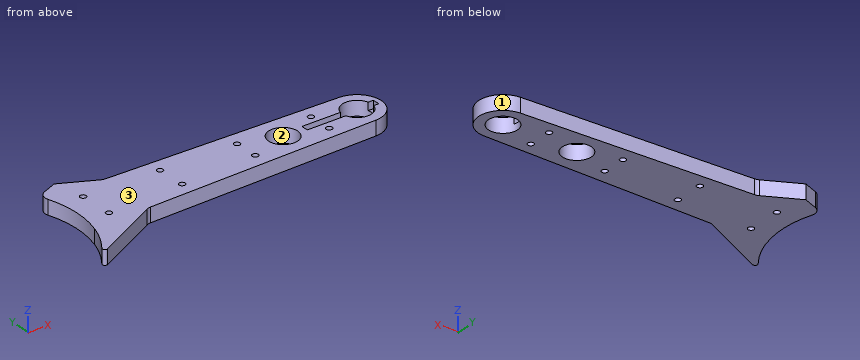
```python
from build123d import *

# Parameters (mm, degrees)
SKETCH1_R                = 13.5
SKETCH1_R_2              = 3
BOSS_EXTRUDE1_DEPTH      = 3
M2_CLEARANCE_HOLE1_D     = 2.4
M2_CLEARANCE_HOLE1_DEPTH = 11.5
CIRPATTERN1_COUNT        = 12
TROU_TARAUD_M1_61_D      = 1.25
ESQUISSE1_R              = 21
ENL_V_MAT_EXTRU_1_DEPTH  = 4
ESQUISSE2_R              = 0.625
ENL_V_MAT_EXTRU_2_DEPTH  = 4
ESQUISSE4_W              = 15
ESQUISSE4_H              = 1.5
ENL_V_MAT_EXTRU_3_DEPTH  = 1.6
ESQUISSE5_R              = 0.625
ENL_V_MAT_EXTRU_4_DEPTH  = 10
BOSS_EXTRU_3_DEPTH       = 3
CONG_2_R                 = 2
CONG_3_R                 = 2
CONG_4_R                 = 0.5


with BuildPart() as part:
    # Sketch1 → Boss-Extrude1 (new body)
    with BuildSketch(Plane.XY):
        with BuildLine():
            Line((18.384776311, 6.5), (80.121567237, 4.998521922))
            ThreePointArc((80.121567237, 4.998521922), (85, 0), (80.121567237, -4.998521922))
            Line((80.121567237, -4.998521922), (18.384776311, -6.5))
            ThreePointArc((18.384776311, -6.5), (-19.5, 0), (18.384776311, 6.5))
        make_face()
        Circle(SKETCH1_R, mode=Mode.SUBTRACT)
        with Locations((64.5, 0)):
            Circle(SKETCH1_R_2, mode=Mode.SUBTRACT)
        with Locations((80, 0)):
            Circle(SKETCH1_R_2, mode=Mode.SUBTRACT)
    extrude(amount=BOSS_EXTRUDE1_DEPTH)

    # M2 Clearance Hole1
    with Locations(Plane.XY.offset(3)):
        with Locations((0, 16.5)):
            m2_clearance_hole1 = Hole(M2_CLEARANCE_HOLE1_D / 2, depth=M2_CLEARANCE_HOLE1_DEPTH)

    # CirPattern1: M2 Clearance Hole1 ×12 about axis
    cirpattern1_axis = Axis((0, 0, 0), (0, 0, 1))
    for i in range(1, CIRPATTERN1_COUNT):
        add(m2_clearance_hole1.rotate(cirpattern1_axis, i * 360 / CIRPATTERN1_COUNT), mode=Mode.SUBTRACT)

    # Trou taraudé M1.61 (through all)
    with Locations(Plane.XY.offset(3)):
        with Locations((56.75, 2.5), (72.25, 2.5), (72.25, -2.5), (56.75, -2.5)):
            Hole(TROU_TARAUD_M1_61_D / 2)

    # Esquisse1 → Enlèv. mat.-Extru.1 (cut, through all)
    with BuildSketch(Plane.XY.offset(3)):
        Circle(ESQUISSE1_R)
    extrude(amount=-ENL_V_MAT_EXTRU_1_DEPTH, mode=Mode.SUBTRACT)

    # Esquisse2 → Enlèv. mat.-Extru.2 (cut, through all)
    with BuildSketch(Plane.XY.offset(3)):
        with Locations((25.251835753, 3.548914074)):
            Circle(ESQUISSE2_R)
        with Locations((25.251835753, -3.548914074)):
            Circle(ESQUISSE2_R)
    extrude(amount=-ENL_V_MAT_EXTRU_2_DEPTH, mode=Mode.SUBTRACT)

    # Esquisse4 → Enlèv. mat.-Extru.3 (cut)
    with BuildSketch(Plane.XY.offset(3)):
        with Locations((76.5, 0)):
            Rectangle(ESQUISSE4_W, ESQUISSE4_H)
    extrude(amount=-ENL_V_MAT_EXTRU_3_DEPTH, mode=Mode.SUBTRACT)

    # Esquisse5 → Enlèv. mat.-Extru.4 (cut)
    with BuildSketch(Plane.XY.offset(3)):
        with Locations((41.000917876, 3.024457037)):
            Circle(ESQUISSE5_R)
        with Locations((41.000917876, -3.024457037)):
            Circle(ESQUISSE5_R)
    extrude(amount=-ENL_V_MAT_EXTRU_4_DEPTH, mode=Mode.SUBTRACT)

    # Esquisse6 → Boss.-Extru.3 (add)
    with BuildSketch(Plane.XY.offset(3)):
        with BuildLine():
            Line((19.981323023, 6.461170967), (31.5, 6.181029406))
            Line((31.5, 6.181029406), (24.077934309, 9.962760764))
            Line((24.077934309, 9.962760764), (19.405232048, 8.027264114))
            ThreePointArc((19.405232048, 8.027264114), (19.708839185, 7.249941929), (19.981323023, 6.461170967))
        make_face()
        with BuildLine():
            Line((15.240466078, -14.489207955), (31.5, -6.181029406))
            Line((31.5, -6.181029406), (20.01179148, -6.460429955))
            ThreePointArc((20.01179148, -6.460429955), (18.077492491, -10.743054438), (15.240466078, -14.489207955))
        make_face()
    extrude(amount=-BOSS_EXTRU_3_DEPTH)

    # Congé2
    cong_2_edges = [part.edges().sort_by_distance(p)[0] for p in [
        (19.405232048, 8.027264114, 1.5),
    ]]
    fillet(cong_2_edges, radius=CONG_2_R)

    # Congé3
    cong_3_edges = [part.edges().sort_by_distance(p)[0] for p in [
        (31.5, 6.181029406, 1.5),
        (31.5, -6.181029406, 1.5),
    ]]
    fillet(cong_3_edges, radius=CONG_3_R)

    # Congé4
    cong_4_edges = [part.edges().sort_by_distance(p)[0] for p in [
        (15.240466078, -14.489207955, 1.5),
    ]]
    fillet(cong_4_edges, radius=CONG_4_R)


solid = part.part
```
Could you check a few things on this model? Use its own coordinates, in mm. Face numbers are marked on the shaded views. Round coordinates to 2 decimals unless told otherwise and drop trailing zeros. Loops run counter-clockwise (first coordinate to the right, second up) from the corner with the lowest first, then second, coordinate; pieces in that order, holes last. Notation, with made-up numbers: M 55.25,56 L 61.25,56 A24 ccw 61.25,66 Z; hole C 65,-3 d5. An arc over 180 degrees is marked long. Write item = value, one per line.
1. I want a section at C-C, the plane x = 72.25. Write out the boundary of the cut face in (y, z) (3 decimals), and give its area (3 significant figures).
Results below:
outline = M -5.19,0 L -3.125,0 L -3.125,3 L -5.19,3 Z; M -1.875,0 L 1.875,0 L 1.875,3 L 0.75,3 L 0.75,1.4 L -0.75,1.4 L -0.75,3 L -1.875,3 Z; M 3.125,0 L 5.19,0 L 5.19,3 L 3.125,3 Z
area = 21.2 mm²
2. I want a section at D-D, the plane z = 0.7. Count the separate pieces of the cut face and the enclosed holes in it, and give its area (3 significant figures).
Results below:
separate_pieces = 1
enclosed_holes = 10
area = 718 mm²
3. Thinking about a two-plate mould opening in Y: for the marked faces 1, 2 and 3, which applies, +Y half, -Y half, draft (parallel to the pull), parting line (faces both ways), or undercut?
Results below:
face_1 = parting line
face_2 = undercut
face_3 = draft
4. I want a section at A-A, the plane y = 0. Write out the boundary of the cut face in (x, z).
Results below:
outline = M 21,0 L 61.5,0 L 61.5,3 L 21,3 Z; M 67.5,0 L 77,0 L 77,1.4 L 69,1.4 L 69,3 L 67.5,3 Z; M 83,0 L 85,0 L 85,3 L 84,3 L 84,1.4 L 83,1.4 Z
5. Will these pins go through, and if not, where does the flat tip stop? P1, Ø1.2, axis at x = 83.5, z = 2.5, coming from the -Y side; P2, Ø1, axis at x = 72.25, y = -2.5, coming from the -Z side; P3, Ø0.8, axis at y = 0, z = 2, coming from the -X side; P4, Ø7, axis at x = 64.5, y = 0, coming from the +Z side.
Results below:
P1 = -4.07
P2 = through
P3 = 21
P4 = 3
6. I want a section at B-B, the plane x = 79.5. Write out the boundary of the cut face in (y, z).
Results below:
outline = M -5.01,0 L -2.96,0 L -2.96,3 L -5.01,3 Z; M 2.96,0 L 5.01,0 L 5.01,3 L 2.96,3 Z
7. I need wall thicknesses on probe 1 along Y at (x, z) = (56.75, 1.7) (3 decimals); probe 2 along Y at (x, z) = (72, 0.45); probe 3 along X at (y, z) = (-0.5, 0.9). Which ranges of each line are inside material? Lowest first, please.
Results below:
probe_1 = -5.567 to -3.125, -1.875 to 1.875, 3.125 to 5.567
probe_2 = -5.2 to -3.07, -1.93 to 1.93, 3.07 to 5.2
probe_3 = 20.99 to 61.54, 67.46 to 77.04, 82.96 to 84.97
